Geometry: see drawing. Coordinates: mm, zero at the bounding-box minimum. Give positions to 0.01 mm unless a question says otherwise; leave off trailing zeros. Write each loop counter-clockwise with the first axis right and the second up, starting at its lowest first coordinate (ties: lowest second). Pieces come first, ordered by that corner, then holes. Notation, with made-up numbers: M 25,13.5 L 48,13.5 A17 ccw 48,44.5 Z; hole C 5,-25.75 d11. An arc over 180 degrees is marked long. Use a Markdown table: item, result. Add a question column.
1) Section B-B on z = 41. Return the cut outline in (x, y), then the cut area to 3 significant figures.
2) Line query: line 1 (Z direction, x = 46.5, y = 0.4) (1 decimal); line 2 (X direction, y = 1.1, z = 41); line 3 (X direction, y = 0.95, z = 32). Output: solid intervals per line, ascending.
3) Pin query (flat end, axial travel): pin 1 (1 mm diameter, centred on x = 33.5, y = 1, fed in from -Z); pin 2 (1 mm diameter, centred on y = 0.5, z = 26, fed in from -X); pin 3 (1 mm diameter, centred on x = 57.5, y = 0.5, fed in from -Z). Return the tip coordinate at first contact, or that it passes through.
4) Section C-C on y = 0.65. Return the cut outline in (x, z).
5) Section A-A on x = 41. Return the cut outline in (y, z).
6) Section D-D on x = 75. Return the cut outline in (y, z).
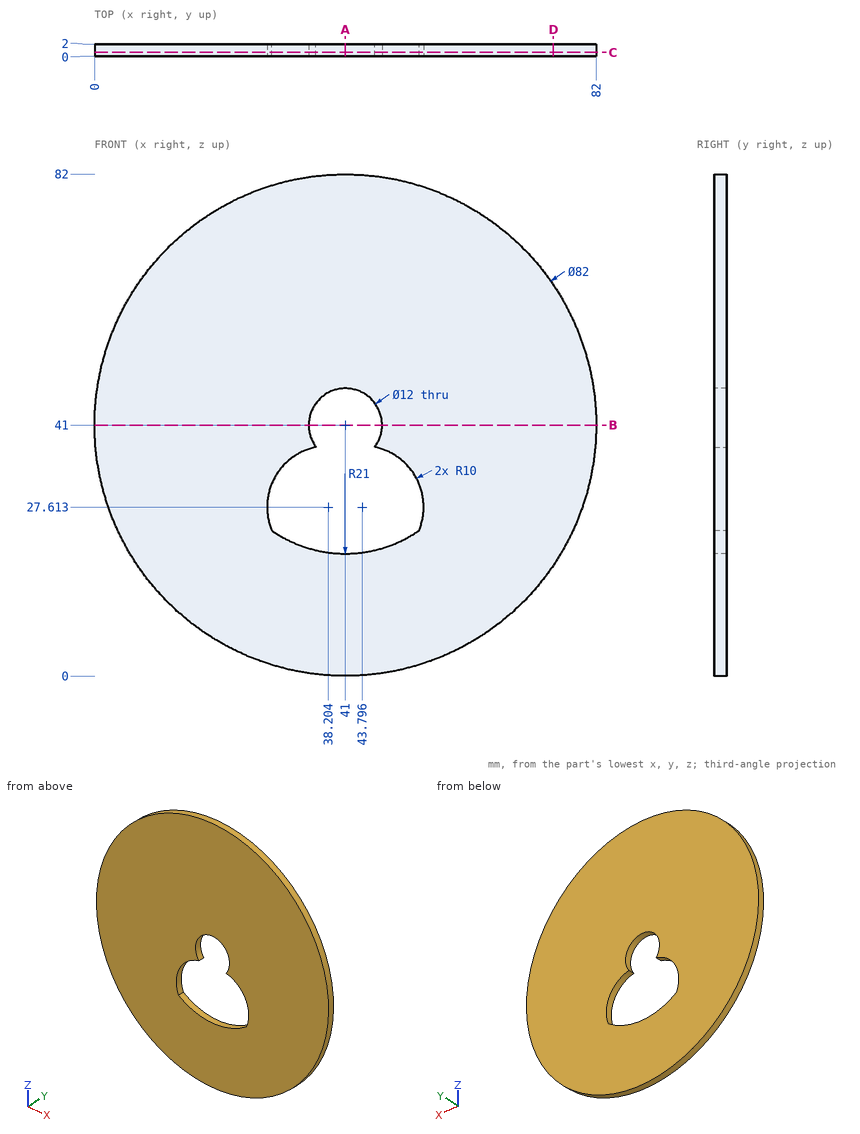
Found:
| question | item | result |
|---|---|---|
| 1 | outline | M 0,0 L 35,0 L 35,2 L 0,2 Z; M 47,0 L 82,0 L 82,2 L 47,2 Z |
| 1 | area | 140 mm² |
| 2 | line 1 | 0.4 to 20.7, 37.2 to 38.6, 43.4 to 81.6 |
| 2 | line 2 | 0 to 35, 47 to 82 |
| 2 | line 3 | 1 to 29.22, 52.78 to 81 |
| 3 | pin 1 | z = 0.6 |
| 3 | pin 2 | x = 2.65 |
| 3 | pin 3 | z = 3.25 |
| 4 | outline | C 41,41 d82; hole M 28.96,23.79 A21 ccw 53.04,23.79 A10 ccw 45.81,37.41 A6 ccw long 36.19,37.41 A10 ccw Z |
| 5 | outline | M 0,0 L 2,0 L 2,20 L 0,20 Z; M 0,47 L 2,47 L 2,82 L 0,82 Z |
| 6 | outline | M 0,18.09 L 2,18.09 L 2,63.91 L 0,63.91 Z |
